Geometry: final body of the model. Coordinates: model frame, mm. Give positions to 0.01 mm unless a question says otherwise; leave off trailing zeros. Loops run counter-clockwise (first coordinate to the right, second up) from the corner with the lowest first, then second, coordinate; pieces in that order, holes last. Notation, with made-up numbers: (82.5, 69.5) - (129.5, 69.5) arc R23 ccw to (129.5, 77.5) - close; hole circle Ø4 at (-33.5, 57). An arc over 180 degrees is marked (long way). Answer in a Markdown table with one row per item.
from build123d import *

# Parameters (mm, degrees)
F7_R      = 29.3293936748
F8_DEPTH  = 9.9209962727
F10_R     = 29.3293936748
F11_DEPTH = 9.9209962727
F13_R     = 29.3293936748
F14_DEPTH = 9.9209962727
F16_R     = 29.3293936748
F17_DEPTH = 9.9209962727
F19_R     = 29.3293936748
F20_DEPTH = 9.9209962727
F22_R     = 29.3293936748
F23_DEPTH = 9.9209962727
F25_R     = 29.3293936748
F26_DEPTH = 9.9209962727
F28_R     = 29.3293936748
F29_DEPTH = 9.9209962727
F31_R     = 29.3293936748
F32_DEPTH = 9.9209962727
F34_R     = 29.3293936748
F35_DEPTH = 9.9209962727
F37_R     = 29.3293936748
F38_DEPTH = 9.9209962727
F40_R     = 29.3293936748
F41_DEPTH = 9.9209962727
F43_R     = 29.3293936748
F44_DEPTH = 9.9209962727
F46_R     = 29.3293936748
F47_DEPTH = 9.9209962727
F49_R     = 29.3293936748
F50_DEPTH = 9.9209962727
F52_R     = 29.3293936748
F53_DEPTH = 9.9209962727
F55_R     = 29.3293936748
F56_DEPTH = 9.9209962727
F58_R     = 29.3293936748
F59_DEPTH = 9.9209962727
F61_R     = 29.3293936748
F64_DEPTH = 9.9209962727
F63_R     = 29.3293936748
F65_DEPTH = 9.9209962727


with BuildPart() as f3:
    # F1 (on Front) → F3 (revolve)
    with BuildSketch(Plane.XZ):
        with BuildLine():
            Line((0, 48.3136710278), (0, -48.3136710278))
            ThreePointArc((0, -48.3136710278), (48.3136710278, 0), (0, 48.3136710278))
        make_face()
    revolve(axis=Axis((0, 0, 56.2952049077), (0, 0, 1)))

    # F7 (on 3pt) → F8 (cut, through all)
    with BuildSketch(Plane(origin=(13.6993544381, 0, 35.8653755428), x_dir=(0.934172359, 0, -0.3568220898), z_dir=(-0.3568220898, 0, -0.934172359))):
        Circle(F7_R)
    extrude(amount=-F8_DEPTH, mode=Mode.SUBTRACT)

    # F10 (on 3pt) → F11 (cut, through all)
    with BuildSketch(Plane(origin=(-13.6993544381, 0, 35.8653755428), x_dir=(0.934172359, 0, 0.3568220898), z_dir=(0.3568220898, 0, -0.934172359))):
        Circle(F10_R)
    extrude(amount=-F11_DEPTH, mode=Mode.SUBTRACT)

    # F13 (on 3pt) → F14 (cut, through all)
    with BuildSketch(Plane(origin=(-22.1660211047, -22.1660211047, 22.1660211047), x_dir=(0.8164965809, -0.4082482905, 0.4082482905), z_dir=(-0.5773502692, -0.5773502692, 0.5773502692))):
        Circle(F13_R)
    extrude(amount=F14_DEPTH, mode=Mode.SUBTRACT)

    # F16 (on 3pt) → F17 (cut, through all)
    with BuildSketch(Plane(origin=(0, -35.8653755428, 13.6993544381), x_dir=(1, 0, 0), z_dir=(0, -0.934172359, 0.3568220898))):
        Circle(F16_R)
    extrude(amount=F17_DEPTH, mode=Mode.SUBTRACT)

    # F19 (on 3pt) → F20 (cut, through all)
    with BuildSketch(Plane(origin=(22.1660211047, -22.1660211047, 22.1660211047), x_dir=(0.8164965809, 0.4082482905, -0.4082482905), z_dir=(0.5773502692, -0.5773502692, 0.5773502692))):
        Circle(F19_R)
    extrude(amount=F20_DEPTH, mode=Mode.SUBTRACT)

    # F22 (on 3pt) → F23 (cut, through all)
    with BuildSketch(Plane(origin=(22.1660211047, 22.1660211047, 22.1660211047), x_dir=(-0.8164965809, 0.4082482905, 0.4082482905), z_dir=(0.5773502692, 0.5773502692, 0.5773502692))):
        Circle(F22_R)
    extrude(amount=F23_DEPTH, mode=Mode.SUBTRACT)

    # F25 (on 3pt) → F26 (cut, through all)
    with BuildSketch(Plane(origin=(0, 35.8653755428, 13.6993544381), x_dir=(1, 0, 0), z_dir=(0, -0.934172359, -0.3568220898))):
        Circle(F25_R)
    extrude(amount=-F26_DEPTH, mode=Mode.SUBTRACT)

    # F28 (on 3pt) → F29 (cut, through all)
    with BuildSketch(Plane(origin=(-22.1660211047, 22.1660211047, 22.1660211047), x_dir=(-0.8164965809, -0.4082482905, -0.4082482905), z_dir=(-0.5773502692, 0.5773502692, 0.5773502692))):
        Circle(F28_R)
    extrude(amount=F29_DEPTH, mode=Mode.SUBTRACT)

    # F31 (on 3pt) → F32 (cut, through all)
    with BuildSketch(Plane(origin=(35.8653755428, -13.6993544381, 0), x_dir=(-0.3568220898, -0.934172359, 0), z_dir=(-0.934172359, 0.3568220898, 0))):
        Circle(F31_R)
    extrude(amount=-F32_DEPTH, mode=Mode.SUBTRACT)

    # F34 (on 3pt) → F35 (cut, through all)
    with BuildSketch(Plane(origin=(35.8653755428, 13.6993544381, 0), x_dir=(0.3568220898, -0.934172359, 0), z_dir=(-0.934172359, -0.3568220898, 0))):
        Circle(F34_R)
    extrude(amount=-F35_DEPTH, mode=Mode.SUBTRACT)

    # F37 (on 3pt) → F38 (cut, through all)
    with BuildSketch(Plane(origin=(-35.8653755428, -13.6993544381, 0), x_dir=(-0.3568220898, 0.934172359, 0), z_dir=(0.934172359, 0.3568220898, 0))):
        Circle(F37_R)
    extrude(amount=-F38_DEPTH, mode=Mode.SUBTRACT)

    # F40 (on 3pt) → F41 (cut, through all)
    with BuildSketch(Plane(origin=(-35.8653755428, 13.6993544381, 0), x_dir=(0.3568220898, 0.934172359, 0), z_dir=(0.934172359, -0.3568220898, 0))):
        Circle(F40_R)
    extrude(amount=-F41_DEPTH, mode=Mode.SUBTRACT)

    # F43 (on 3pt) → F44 (cut, through all)
    with BuildSketch(Plane(origin=(-22.1660211047, 22.1660211047, -22.1660211047), x_dir=(0.8164965809, 0.4082482905, -0.4082482905), z_dir=(0.5773502692, -0.5773502692, 0.5773502692))):
        Circle(F43_R)
    extrude(amount=-F44_DEPTH, mode=Mode.SUBTRACT)

    # F46 (on 3pt) → F47 (cut, through all)
    with BuildSketch(Plane(origin=(0, 35.8653755428, -13.6993544381), x_dir=(1, 0, 0), z_dir=(0, -0.934172359, 0.3568220898))):
        Circle(F46_R)
    extrude(amount=-F47_DEPTH, mode=Mode.SUBTRACT)

    # F49 (on 3pt) → F50 (cut, through all)
    with BuildSketch(Plane(origin=(22.1660211047, 22.1660211047, -22.1660211047), x_dir=(0.8164965809, -0.4082482905, 0.4082482905), z_dir=(-0.5773502692, -0.5773502692, 0.5773502692))):
        Circle(F49_R)
    extrude(amount=-F50_DEPTH, mode=Mode.SUBTRACT)

    # F52 (on 3pt) → F53 (cut, through all)
    with BuildSketch(Plane(origin=(22.1660211047, -22.1660211047, -22.1660211047), x_dir=(-0.8164965809, -0.4082482905, -0.4082482905), z_dir=(-0.5773502692, 0.5773502692, 0.5773502692))):
        Circle(F52_R)
    extrude(amount=-F53_DEPTH, mode=Mode.SUBTRACT)

    # F55 (on 3pt) → F56 (cut, through all)
    with BuildSketch(Plane(origin=(13.6993544381, 0, -35.8653755428), x_dir=(0.934172359, 0, 0.3568220898), z_dir=(-0.3568220898, 0, 0.934172359))):
        Circle(F55_R)
    extrude(amount=-F56_DEPTH, mode=Mode.SUBTRACT)

    # F58 (on 3pt) → F59 (cut, through all)
    with BuildSketch(Plane(origin=(0, -35.8653755428, -13.6993544381), x_dir=(-1, 0, 0), z_dir=(0, 0.934172359, 0.3568220898))):
        Circle(F58_R)
    extrude(amount=-F59_DEPTH, mode=Mode.SUBTRACT)

    # F61 (on 3pt) → F64 (cut, through all)
    with BuildSketch(Plane(origin=(-13.6993544381, 0, -35.8653755428), x_dir=(0.934172359, 0, -0.3568220898), z_dir=(0.3568220898, 0, 0.934172359))):
        Circle(F61_R)
    extrude(amount=-F64_DEPTH, mode=Mode.SUBTRACT)

    # F63 (on 3pt) → F65 (cut, through all)
    with BuildSketch(Plane(origin=(-22.1660211047, -22.1660211047, -22.1660211047), x_dir=(0.8164965809, -0.4082482905, -0.4082482905), z_dir=(-0.5773502692, -0.5773502692, -0.5773502692))):
        Circle(F63_R)
    extrude(amount=F65_DEPTH, mode=Mode.SUBTRACT)


solid = f3.part
Q1. Cut plane A-A (y = 14.5). Output: boundary loops of the cut face in (x, z).
Check values:
| item | result |
|---|---|
| outline | (-35.56, -16.44) - (-17.64, -34.36) - (0, -41.1) - (17.64, -34.36) - (35.56, -16.44) - (35.56, 16.44) - (17.64, 34.36) - (0, 41.1) - (-17.64, 34.36) - (-35.56, 16.44) - close |
Q2. Material intervals for line 1 along Z through (x, y) = (17, -14.5); line 2 along Z through (x, y) = (-4.5, 20); line 3 along Y through (x, z) = (-22, -8.5), sorted ascending.
Check values:
| item | result |
|---|---|
| line 1 | -34.6 to 34.6 |
| line 2 | -39.38 to 39.38 |
| line 3 | -36 to 36 |
Q3. Cut plane D-D (x = -27.5). Output: boundary loops of the cut face in (y, z), and give its area (3 significant figures).
Check values:
| item | result |
|---|---|
| outline | (-35.6, -3.4) - (-8.4, -30.59) - (8.4, -30.59) - (35.6, -3.4) - (35.6, 3.4) - (8.4, 30.59) - (-8.4, 30.59) - (-35.6, 3.4) - close |
| area | 2,880 mm² |
Q4. First-contact query: pin 1 (10 mm diameter, centred on x = 28.5, z = 15, fed in from -Y); pin 2 (10 mm diameter, centred on x = 15, y = -22, fed in from +Z); pin 3 (4 mm diameter, centred on x = -20, y = -19.5, fed in from -Z). Flat tips, straight axial feed; report the tip coordinate or a pass-through.
Check values:
| item | result |
|---|---|
| pin 1 | y = -30.07 |
| pin 2 | z = 36.57 |
| pin 3 | z = -29.83 |
Q5. Cut plane C-C (z = 18). Output: boundary loops of the cut face in (x, y), and give its area (3 significant figures).
Check values:
| item | result |
|---|---|
| outline | (-41.1, 0) - (-36.52, -11.97) - (-14.28, -34.22) - (14.28, -34.22) - (36.52, -11.97) - (41.1, 0) - (36.52, 11.97) - (14.28, 34.22) - (-14.28, 34.22) - (-36.52, 11.97) - close |
| area | 4,120 mm² |
Q6. Cut plane B-B (x = 34.5). Output: boundary loops of the cut face in (y, z).
Check values:
| item | result |
|---|---|
| outline | (-17.27, -14.72) - (-4.08, -27.92) - (4.08, -27.92) - (17.27, -14.72) - (17.27, 14.72) - (4.08, 27.92) - (-4.08, 27.92) - (-17.27, 14.72) - close |
